from build123d import *

# Parameters (mm, degrees)
F1_DEPTH = 350


with BuildPart() as f1:
    # F0 (on Top) → F1 (new body)
    with BuildSketch(Plane.XY):
        Polygon((102.266435, -45.12095), (-97.733565, -45.12095), (-97.733565, -80.12095), (-77.733565, -80.12095), (-77.733565, -76.62095), (-52.733565, -76.62095), (-52.733565, -80.12095), (-32.733565, -80.12095), (-32.733565, -76.62095), (7.266435, -76.62095), (7.266435, -80.12095), (32.266435, -80.12095), (32.266435, -76.62095), (92.266435, -76.62095), (92.266435, -80.12095), (102.266435, -80.12095), align=None)
    extrude(amount=-F1_DEPTH)


solid = f1.part
Geometry: final body of the model. Coordinates: model frame, mm. A direction names the side the tool comes from. Round coordinates to 2 decimals unless told otherwise and drop trailing zeros. Loops run counter-clockwise (first coordinate to the right, second up) from the corner with the lowest first, then second, coordinate; pieces in that order, holes last. Notation, with made-up numbers: (15, 54) -> (28, 54) arc R10 cw to (28, 68) -> close; hole circle Ø3 at (28, -37.5). An arc over 180 degrees is marked (long way). One line per question, with ' | ' between items. Start each with the question number.
1. Contact query for a flat-ended pin moving along its axis: pin 1 (10 mm diameter, centred on x = 70.5, z = -113, fed in from -Y). Output: stop coordinate, or through.
2. Section B-B on x = 73. Output: boundary loops of the cut face in (y, z), and give its area (3 significant figures).
3. Mould query, pull axis X, two halves, no side actions, for faces 1 (the face through (62, -76.621, -173)), 2 (the face through (102.266, -63, -173)), 3 (the face through (-43, -80.121, -173)). Classes: pulls with the +X half, pulls with the -X half, needs draft (parallel to the pull), parting line crosses it, or undercut.
4. Set-up query: faces 4 (the face through (-65, -76.621, -173)), 5 (the face through (-88, -80.121, -173)). Return all of +Z, -Z, +X, -X, +Y, -Y with unobstructed straight access to the full face (end or side cutting, diameter ignored); none if empty.
5. Line query: line 1 along X through (y, z) = (-77, -314.5); line 2 along Y through (x, z) = (80.5, -71). Output: solid intervals per line, ascending. Write a range as [from, to].
6. Section A-A on z = -285. Output: boundary loops of the cut face in (x, y), and give its area (3 significant figures).
Returned:
1) pin 1: stops at y = -76.62
2) outline: (-76.62, -350) -> (-45.12, -350) -> (-45.12, 0) -> (-76.62, 0) -> close | area: 11,000 mm2
3) face 1: undercut | face 2: pulls with the +X half | face 3: needs draft
4) face 4: +Z, -Z, -Y | face 5: +Z, -Z, +X, -X, -Y
5) line 1: x = [-97.73, -77.73], [-52.73, -32.73], [7.27, 32.27], [92.27, 102.27] | line 2: y = [-76.62, -45.12]
6) outline: (-97.73, -80.12) -> (-77.73, -80.12) -> (-77.73, -76.62) -> (-52.73, -76.62) -> (-52.73, -80.12) -> (-32.73, -80.12) -> (-32.73, -76.62) -> (7.27, -76.62) -> (7.27, -80.12) -> (32.27, -80.12) -> (32.27, -76.62) -> (92.27, -76.62) -> (92.27, -80.12) -> (102.27, -80.12) -> (102.27, -45.12) -> (-97.73, -45.12) -> close | area: 6,560 mm2
